Geometry: see drawing. Coordinates: mm, zero at the bounding-box minimum. A direction names the side the tool comes from. Coordinates: 2 decimals unless noted, no trailing zeros. Order: outer loops, then holes, each group sorted by start corner. A loop starts at its lowest first (then second) coordinate and runs counter-clockwise, first axis right, second up.
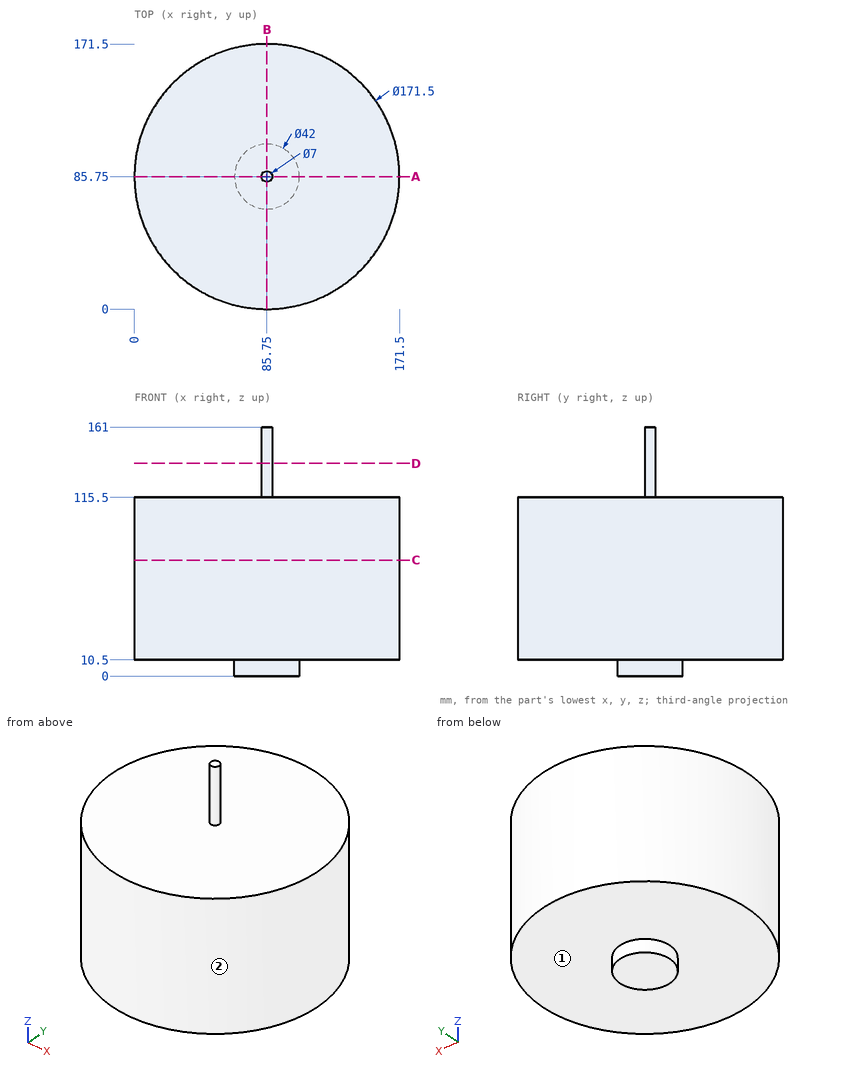
Q1. Section query D-D on z = 137.5. Output: boundary loops of the cut face in (x, y).
Solutions:
outline: circle Ø7 at (85.75, 85.75)
Q2. Material intervals for line 1 along Z through (x, y) = (51, 128); line 2 along Z through (x, y) = (87.5, 101); line 3 along Y through (x, z) = (116, 79), sorted ascending.
Solutions:
line 1: z = 10.5 to 115.5
line 2: z = 0 to 115.5
line 3: y = 5.51 to 165.99
Q3. Section query A-A on y = 85.75. Output: boundary loops of the cut face in (x, z).
Solutions:
outline: (0, 10.5) - (64.75, 10.5) - (64.75, 0) - (106.75, 0) - (106.75, 10.5) - (171.5, 10.5) - (171.5, 115.5) - (89.25, 115.5) - (89.25, 161) - (82.25, 161) - (82.25, 115.5) - (0, 115.5) - close
Q4. Section query C-C on z = 75. Output: boundary loops of the cut face in (x, y).
Solutions:
outline: circle Ø171.5 at (85.75, 85.75)
Q5. Set-up query: the marked faces 1 and 2. Return all of +Z, -Z, +X, -X, +Y, -Y with unobstructed straight access to the full face (end or side cutting, diameter ignored); none if empty.
Solutions:
face 1: -Z
face 2: +Z, -Z
Q6. Pin query (flat end, axial travel): P1, Ø3, axis at x = 119.5, y = 37, coming from the +Z side; P2, Ø3, axis at x = 82.5, z = 120, coming from the -Y side; P3, Ø1.5, axis at x = 72, z = 78, coming from the -Y side. Return the tip coordinate at first contact, or that it passes through.
Solutions:
P1: stops at z = 115.5
P2: stops at y = 82.72
P3: stops at y = 0.99
